from build123d import *

# Parameters (mm, degrees)
SKETCH1_W                            = 120
SKETCH1_H                            = 90
BOSS_EXTRUDE1_DEPTH                  = 3
CHAMFER1_SIZE                        = 5
F_3_0_3_DIAMETER_HOLE2_D             = 3
MIRROR1_AT_THE_SECOND_PLANE_COPY_1_D = 3
F_3_0_3_DIAMETER_HOLE3_D             = 3
F_5_0_5_DIAMETER_HOLE1_D             = 5
SKETCH11_W                           = 15
SKETCH11_H                           = 20
CUT_EXTRUDE1_DEPTH                   = 76.059976019
CHAMFER2_SIZE                        = 3


with BuildPart() as part:
    # Sketch1 → Boss-Extrude1 (new body)
    with BuildSketch(Plane(origin=(0, 0, 0), x_dir=(1, 0, 0), z_dir=(0, 1, 0))):
        Rectangle(SKETCH1_W, SKETCH1_H)
    extrude(amount=BOSS_EXTRUDE1_DEPTH)

    # Chamfer1
    chamfer1_edges = [part.edges().sort_by_distance(p)[0] for p in [
        (60, 1.5, 45),
        (-60, 1.5, 45),
        (-60, 1.5, -45),
        (60, 1.5, -45),
    ]]
    chamfer(chamfer1_edges, length=CHAMFER1_SIZE)

    # Ø3.0 (3) Diameter Hole2 (through all)
    with Locations(Plane.XZ):
        with Locations((-51.843145751, 36.843145751)):
            f_3_0_3_diameter_hole2 = Hole(F_3_0_3_DIAMETER_HOLE2_D / 2)

    # Mirror1: Ø3.0 (3) Diameter Hole2 across plane
    add(f_3_0_3_diameter_hole2.mirror(Plane.XY), mode=Mode.SUBTRACT)

    # Mirror1 at the second plane: Ø3.0 (3) Diameter Hole2 across plane
    add(f_3_0_3_diameter_hole2.mirror(Plane(origin=(0, 0, 0), x_dir=(0, 0, 1), z_dir=(1, 0, 0))), mode=Mode.SUBTRACT)

    # Mirror1 at the second plane copy 1 (through all)
    with Locations(Plane(origin=(0, 0, 0), x_dir=(-1, 0, 0), z_dir=(0, -1, 0))):
        with Locations((-51.843145751, 36.843145751)):
            Hole(MIRROR1_AT_THE_SECOND_PLANE_COPY_1_D / 2)

    # Ø3.0 (3) Diameter Hole3 (through all)
    with Locations(Plane(origin=(0, 3, 0), x_dir=(1, 0, 0), z_dir=(0, 1, 0))):
        with Locations((46, -13.462985276), (53, -13.462985276), (46, 13.462985276), (53, 13.462985276), (13.462985276, -31), (13.462985276, -38), (-13.462985276, -38), (-13.462985276, -31), (-46, -13.462985276), (-53, -13.462985276), (-46, 13.462985276), (-53, 13.462985276), (13.462985276, 31), (13.462985276, 38), (-13.462985276, 31), (-13.462985276, 38)):
            Hole(F_3_0_3_DIAMETER_HOLE3_D / 2)

    # Ø5.0 (5) Diameter Hole1 (through all)
    with Locations(Plane(origin=(0, 0, 0), x_dir=(-1, 0, 0), z_dir=(0, -1, 0))):
        with Locations((-35, 0)):
            Hole(F_5_0_5_DIAMETER_HOLE1_D / 2)

    # Sketch11 → Cut-Extrude1 (cut, through all)
    with BuildSketch(Plane(origin=(0, 0, 0), x_dir=(-1, 0, 0), z_dir=(0, -1, 0))):
        with Locations((27.5, 0)):
            Rectangle(SKETCH11_W, SKETCH11_H)
    extrude(amount=-CUT_EXTRUDE1_DEPTH, mode=Mode.SUBTRACT)

    # Chamfer2
    chamfer2_edges = [part.edges().sort_by_distance(p)[0] for p in [
        (-35, 1.5, -10),
        (-35, 1.5, 10),
        (-20, 1.5, 10),
        (-20, 1.5, -10),
    ]]
    chamfer(chamfer2_edges, length=CHAMFER2_SIZE)


solid = part.part
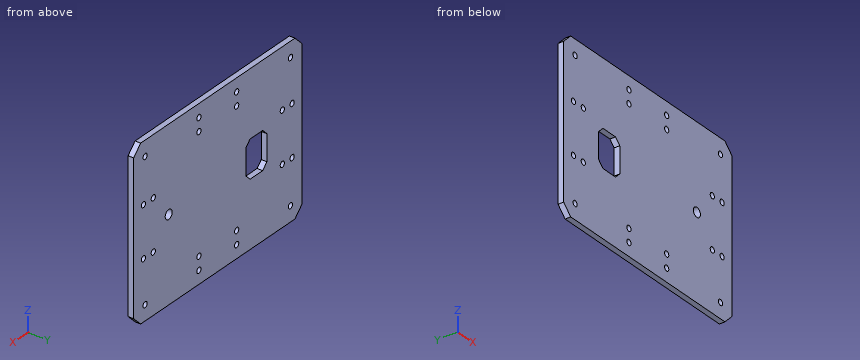
Geometry check sheet. Reference: the model listing, model coordinates, mm. Give positions to 0.01 mm unless a question says otherwise; leave off trailing zeros. Write each loop counter-clockwise with the first axis right and the second up, starting at its lowest first coordinate (ties: lowest second). Pieces come first, ordered by that corner, then holes.
1) Cross-section at D-D (z = -5.5). Record the boundary of the cut face in (x, y).
Values follow:
outline: (-60, 0) - (-35, 0) - (-35, 3) - (-60, 3) - close; (-20, 0) - (60, 0) - (60, 3) - (-20, 3) - close
2) Thickness scan on line 1 (Z direction, x = 46, y = 0.95); line 2 (X direction, y = 1.45, z = 13.5); line 3 (X direction, y = 1, z = -31). Record the ranges inside material, lowest first.
Values follow:
line 1: z = -45 to -14.96, -11.96 to 11.96, 14.96 to 45
line 2: x = -60 to -54.5, -51.5 to -47.5, -44.5 to 44.5, 47.5 to 51.5, 54.5 to 60
line 3: x = -60 to -14.96, -11.96 to 11.96, 14.96 to 60
3) Cross-section at C-C (x = -46). Record the boundary of the cut face in (y, z), plus the area to 3 significant figures.
Values follow:
outline: (0, -45) - (3, -45) - (3, -14.96) - (0, -14.96) - close; (0, -11.96) - (3, -11.96) - (3, 11.96) - (0, 11.96) - close; (0, 14.96) - (3, 14.96) - (3, 45) - (0, 45) - close
area: 252 mm2
4) Go/stop test with a flat-tipped pin: pin 1 Ø2.5 at (x, z) = (-51.84, -36.84) entering from +Y. Record where the tip stops, or that it passes through.
Values follow:
pin 1: passes through
5) Cross-section at B-B (z = 31). Record the boundary of the cut face in (x, y), plus the area to 3 significant figures.
Values follow:
outline: (-60, 0) - (-14.96, 0) - (-14.96, 3) - (-60, 3) - close; (-11.96, 0) - (11.96, 0) - (11.96, 3) - (-11.96, 3) - close; (14.96, 0) - (60, 0) - (60, 3) - (14.96, 3) - close
area: 342 mm2
6) Cross-section at A-A (x = 35). Record the boundary of the cut face in (y, z).
Values follow:
outline: (0, -45) - (3, -45) - (3, -2.5) - (0, -2.5) - close; (0, 2.5) - (3, 2.5) - (3, 45) - (0, 45) - close
